Source: CAD feature listing. Evaluate the final solid. Frame: model axes, mm. A direction names the side the tool comes from. Round coordinates to 2 decimals unless told otherwise and drop trailing zeros. Loops run counter-clockwise (first coordinate to the right, second up) from the corner with the lowest first, then second, coordinate; pieces in that order, holes last.
(1) Section C-C, the plane z = 114. Return the cut outline in (x, y), plus the area to 3 significant figures.
(2) Set-up query: faces 1 (the flat face through (0, 0, 0)), 2 (the cylindrical face through (-0.54, -2.44, 10.11)), 3 (the cylindrical face through (-0.54, -2.44, 152.39)). Return all of +Z, -Z, +X, -X, +Y, -Y with unobstructed straight access to the full face (end or side cutting, diameter ignored); none if empty.
(3) Section A-A, the plane x = 0. Return the cut outline in (y, z), plus the area to 3 significant figures.
(4) First-contact query: pin 1 Ø1 at (y, z) = (-2.5, 29) entering from -X. Flat tip, straight axial feed; report the tip coordinate or a pass-through.
(5) Material intervals for probe 1 along Z at (x, y) = (1.75, -1); probe 2 along Z at (x, y) = (0.5, 2.5); probe 3 along X at (y, z) = (0.25, 59.5), sorted ascending.
```python
from build123d import *

# Parameters (mm, degrees)
F0_R     = 4
F1_DEPTH = 155.6
F2_R     = 6.5
F2_R_2   = 2.5
F3_DEPTH = 20
F4_R     = 4
F4_R_2   = 2.5
F5_DEPTH = 6
F6_SIZE  = 0.5


with BuildPart() as f1:
    # F0 (on Top) → F1 (new body)
    with BuildSketch(Plane.XY):
        Circle(F0_R)
    extrude(amount=F1_DEPTH)

    # F2 (on Top) → F3 (cut)
    with BuildSketch(Plane.XY):
        Circle(F2_R)
        Circle(F2_R_2, mode=Mode.SUBTRACT)
    extrude(amount=F3_DEPTH, mode=Mode.SUBTRACT)

    # F4 (on face) → F5 (cut)
    with BuildSketch(Plane.XY.offset(155.6)):
        Circle(F4_R)
        Circle(F4_R_2, mode=Mode.SUBTRACT)
    extrude(amount=-F5_DEPTH, mode=Mode.SUBTRACT)

    # F6
    f6_edges = [f1.edges().sort_by_distance(p)[0] for p in [
        (-2.5, 0, 0),
        (-4, 0, 20),
        (-4, 0, 149.6),
        (-2.5, 0, 155.6),
    ]]
    chamfer(f6_edges, length=F6_SIZE)


solid = f1.part
```
Output values:
1. outline: circle Ø8 at (0, 0)
1. area: 50.3 mm2
2. face 1: -Z, +X, -X, +Y, -Y
2. face 2: -Z
2. face 3: +Z
3. outline: (-4, 20.5) - (-3.5, 20) - (-2.5, 20) - (-2.5, 0.5) - (-2, 0) - (2, 0) - (2.5, 0.5) - (2.5, 20) - (3.5, 20) - (4, 20.5) - (4, 149.1) - (3.5, 149.6) - (2.5, 149.6) - (2.5, 155.1) - (2, 155.6) - (-2, 155.6) - (-2.5, 155.1) - (-2.5, 149.6) - (-3.5, 149.6) - (-4, 149.1) - close
3. area: 1,170 mm2
4. pin 1: stops at x = -3.46
5. probe 1: z = 0.02 to 155.58
5. probe 2: z = 20 to 149.6
5. probe 3: x = -3.99 to 3.99
